from build123d import *

# Parameters (mm, degrees)
F1_DEPTH = 15


with BuildPart() as f1:
    # F0 (on Top) → F1 (new body)
    with BuildSketch(Plane.XY):
        Polygon((-11, 0), (0, 0), (0, 3), (-4, 3), (-6, 3), (-9.5, 3), (-9.5, 6.5), (-7.4, 6.5), (-7.4, 8.6), (-11, 8.6), (-12, 8.6), (-12, 0), align=None)
    extrude(amount=F1_DEPTH)

    # F2: F1 across plane


with BuildPart() as f1_1:
    add(f1.part)
    add(f1.part.mirror(Plane.YZ))


solid = f1_1.part
Verification items for the finished model (mm, model axes). A direction names the side the tool comes from. Give positions to 0.01 mm unless a question says otherwise; leave off trailing zeros. Write each loop counter-clockwise with the first axis right and the second up, starting at its lowest first coordinate (ties: lowest second). Pieces come first, ordered by that corner, then holes. Notation, with made-up numbers: M 86,-16.5 L 136,-16.5 A31 cw 136,14.5 Z; hole C 20,-16.5 d7. An arc over 180 degrees is marked long. Put each result on its own line as item: value. Start each with the question number.
1. Set-up check for faces 4 (the face through (-7.4, 8, 7)), 5 (the face through (0, 0, 7)), 6 (the face through (-8, 6.5, 7)): record each of +Z, -Z, +X, -X, +Y, -Y from which the full face is reachable in a straight line by a thin tool's end or side.
2. Section check D-D (x = -0.5). Record the cut outline in (y, z).
3. Draft check along X on faces 1 (the face through (7.4, 8, 7)), 2 (the face through (-12, 4, 7)), 3 (the face through (10, 8.6, 7)). Enter one of: +X half, -X half, draft (parallel to the pull), parting line (faces both ways), or undercut.
4. Go/stop test with a flat-tipped pin: pin 1 Ø1.5 at (x, y) = (-9, 5.5) entering from +Z. Record where the tip stops, or that it passes through.
5. Section check A-A (y = 7.25). Record the cut outline in (x, z).
6. Scan lines: line 1 along X through (y, z) = (3.25, 13.5); line 2 along Y through (x, z) = (8.5, 5); line 3 along X through (y, z) = (7.25, 3.5). Record each from-to range of solid material in increasing order. Write a range as [from, to].
7. Section check B-B (z = 11.75). Record the cut outline in (x, y), and give its area (3 significant figures).
8. Section check C-C (y = 3.75). Record the cut outline in (x, z).
Answer list:
1. face 4: +Z, -Z, +Y
1. face 5: +Z, -Z, +X, -X, -Y
1. face 6: +Z, -Z
2. outline: M 0,0 L 3,0 L 3,15 L 0,15 Z
3. face 1: undercut
3. face 2: -X half
3. face 3: draft
4. pin 1: z = 15
5. outline: M -12,0 L -7.4,0 L -7.4,15 L -12,15 Z; M 7.4,0 L 12,0 L 12,15 L 7.4,15 Z
6. line 1: [-12, -9.5], [9.5, 12]
6. line 2: [0, 3], [6.5, 8.6]
6. line 3: [-12, -7.4], [7.4, 12]
7. outline: M -12,0 L 12,0 L 12,8.6 L 7.4,8.6 L 7.4,6.5 L 9.5,6.5 L 9.5,3 L -9.5,3 L -9.5,6.5 L -7.4,6.5 L -7.4,8.6 L -12,8.6 Z
7. area: 109 mm2
8. outline: M -12,0 L -9.5,0 L -9.5,15 L -12,15 Z; M 9.5,0 L 12,0 L 12,15 L 9.5,15 Z
